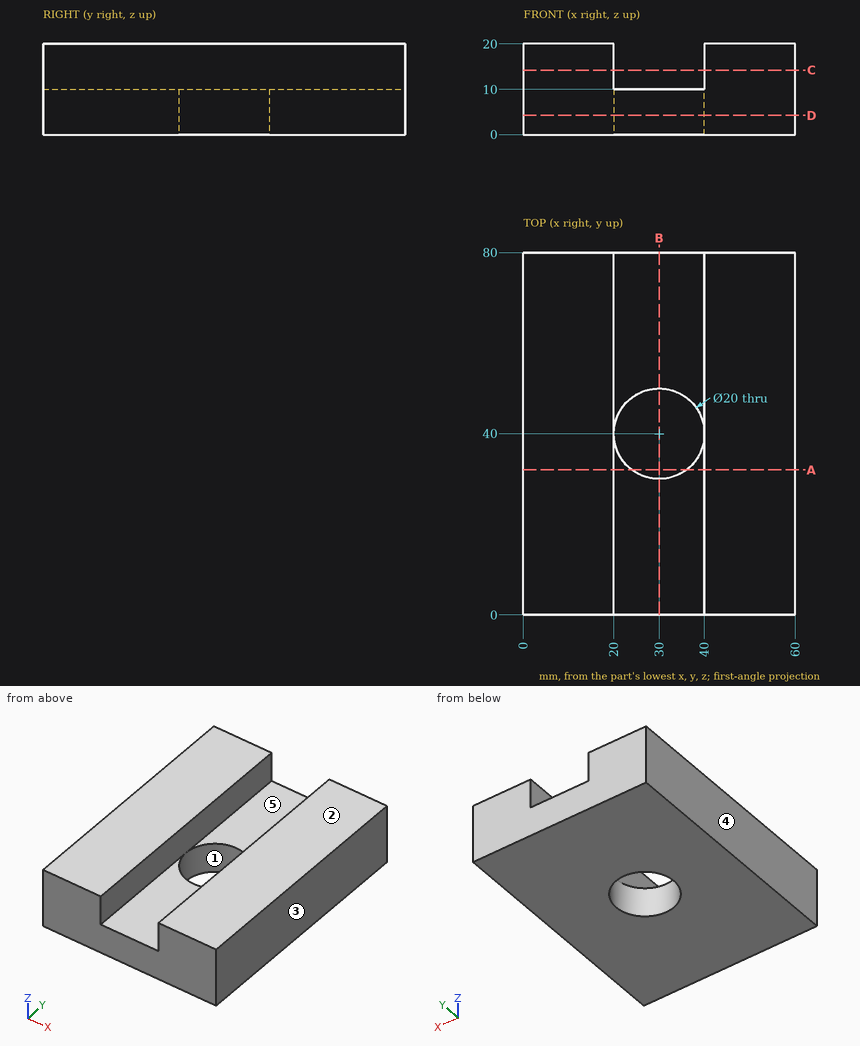
For this review, use the dimensioned drawing (mm, ordinates from the lowest corner) and the shaded views. A direction names the side the tool comes from. Give positions to 0.01 mm unless a question says otherwise; leave off trailing zeros. Order: outer loops, then holes, each group sorted by start corner. A loop starts at its lowest first (then second) coordinate and runs counter-clockwise, first axis right, second up. Notation, with made-up numbers: (71.25, 48) - (126.25, 48) arc R21 cw to (126.25, 78) - close; hole circle Ø10 at (2, 31). An arc over 180 degrees is marked (long way). Use CSV: the item, a comma, the result in double quotes. Start each with the question number.
Q1. Take a section at A-A (y = 32). State the section outline as (x, z) points.
Q2. Draft analysis for pull direction X (two halves, no side actions). For the marked faces 1, 2 and 3, state which applies: pulls with the +X half, pulls with the -X half, needs draft (parallel to the pull), parting line crosses it, or undercut.
Q3. Machinability: for the marked faces 4 and 5, which of the approach directions +Z, -Z, +X, -X, +Y, -Y give a long, thin tool a straight path to every point of the face, cutting with its end or side? Answer none if there is none.
Q4. Take a section at D-D (z = 4.25). State the section outline as (x, y) points.
Q5. For line 1 (X direction, y = 40, z = 7.25); line 2 (Y direction, x = 30, z = 4); line 3 (Z direction, x = 31, y = 69), list the stretches that pass through material, from the lowest coordinate up.
Q6. Take a section at C-C (z = 14.25). State the section outline as (x, y) points.
Q7. Take a section at B-B (x = 30). State the section outline as (y, z) points, and give its area (3 significant figures).
Calculated:
1,outline,"(0, 0) - (24, 0) - (24, 10) - (20, 10) - (20, 20) - (0, 20) - close; (36, 0) - (60, 0) - (60, 20) - (40, 20) - (40, 10) - (36, 10) - close"
2,face 1,"undercut"
2,face 2,"needs draft"
2,face 3,"pulls with the +X half"
3,face 4,"+Z, -Z, -X, +Y, -Y"
3,face 5,"+Z, +Y, -Y"
4,outline,"(0, 0) - (60, 0) - (60, 80) - (0, 80) - close; hole circle Ø20 at (30, 40)"
5,line 1,"x = 0 to 20, 40 to 60"
5,line 2,"y = 0 to 30, 50 to 80"
5,line 3,"z = 0 to 10"
6,outline,"(0, 0) - (20, 0) - (20, 80) - (0, 80) - close; (40, 0) - (60, 0) - (60, 80) - (40, 80) - close"
7,outline,"(0, 0) - (30, 0) - (30, 10) - (0, 10) - close; (50, 0) - (80, 0) - (80, 10) - (50, 10) - close"
7,area,"600 mm²"
